CAD build for the part. Positions are in the model's coordinates, mm. A direction names the side the tool comes from. Round coordinates to 2 decimals unless told otherwise and drop trailing zeros. Loops run counter-clockwise (first coordinate to the right, second up) from the corner with the lowest first, then second, coordinate; pieces in that order, holes last.
```python
from build123d import *

# Parameters (mm, degrees)
F1_DEPTH = 17
F2_T     = 1
F3_R     = 3.5616299701
F3_R_2   = 3.3888359299
F3_R_3   = 3.7011523773
F3_R_4   = 3.561628653
F4_DEPTH = 25


with BuildPart() as f1:
    # F0 (on Top) → F1 (new body)
    with BuildSketch(Plane.XY):
        Polygon((-43.5885637999, 51.4345057309), (-45.7195602357, 49.4972355664), (-45.7195602357, -35.3551693261), (-43.7822900712, -37.6798920333), (41.6512936354, -37.6798920333), (43.5885637999, -35.5488955975), (43.5885637999, 49.303509295), (41.8450199068, 51.4345057309), align=None)
        Polygon((-9.6863470972, -24.5064590126), (-9.8800742999, -12.882841751), (7.9428050667, -12.882841751), (7.9428050667, -24.5064590126), align=None, mode=Mode.SUBTRACT)
        Polygon((-29.2527694255, 31.4806289971), (-21.6974187642, 39.2297059298), (19.7601504624, 39.4234322011), (27.315499261, 31.2869027257), (27.315499261, 10.364391841), (19.7601504624, 3.3902216237), (9.6863470972, 3.3902216237), (8.3302585408, 1.6466790112), (8.3302585408, -8.8145760819), (-9.6863470972, -8.8145760819), (-9.6863470972, 6.6835791804), (-2.3247229401, 14.4326565787), (10.4612540454, 14.4326565787), (10.4612540454, 26.2500010431), (8.5239848122, 27.9935430735), (-11.817343533, 27.9935430735), (-11.817343533, 26.4437273145), (-11.817343533, 15.0138381869), (-29.2527694255, 15.0138381869), align=None, mode=Mode.SUBTRACT)
    extrude(amount=F1_DEPTH)

    # F2
    f2_openings = [f1.faces().sort_by_distance(p)[0] for p in [
        (-0.871772, 50.172867, 17),
    ]]
    offset(amount=F2_T, openings=f2_openings, kind=Kind.INTERSECTION)

    # F3 (on Top) → F4 (cut)
    with BuildSketch(Plane.XY):
        with Locations((35.9209813178, 43.8607819378)):
            Circle(F3_R)
        with Locations((-37.6952588558, 43.4733256698)):
            Circle(F3_R_2)
        with Locations((35.9209813178, -29.5617301017)):
            Circle(F3_R_3)
        with Locations((-37.8889851272, -29.5617301017)):
            Circle(F3_R_4)
    extrude(amount=-F4_DEPTH, mode=Mode.SUBTRACT)


solid = f1.part
```
Item 1: Cut at B-B, the plane z = 4. State how many separate pieces and enclosed holes the cut face has, plus the area to 3 significant figures.
Answers follow:
separate pieces: 3
enclosed holes: 3
area: 662 mm2
Item 2: Probe line 1 (Y direction, x = 18, z = 1); line 2 (X direction, y = 0.5, z = 5.5); line 3 (Y direction, x = -29.5, z = 7.75). List the from-to ranges inside material, lowest first.
Answers follow:
line 1: y = -38.68 to -37.68, 3.39 to 4.39, 38.42 to 39.42, 51.43 to 52.43
line 2: x = -46.72 to -45.72, -9.69 to -8.69, 7.33 to 8.33, 43.59 to 44.59
line 3: y = -38.68 to -37.68, 51.43 to 52.43
Item 3: Two-plate mould, pull along X, no slides. Class faces 4 (the flat face through (14, 4.39, 8)), 5 (the flat face through (43.32, -37.33, 7.87)), 6 (the flat face through (22.89, 7.64, 7.87)), 7 (the flat face through (-12, 8, -1)): released by +X, released by -X, zero draft, split by the parting line, or undercut.
Answers follow:
face 4: undercut
face 5: released by +X
face 6: undercut
face 7: zero draft
Item 4: Cut at A-A, the plane y = 19. Give the cut face in (x, z).
Answers follow:
outline: (-46.72, -1) - (-28.25, -1) - (-28.25, 17) - (-29.25, 17) - (-29.25, 0) - (-45.72, 0) - (-45.72, 17) - (-46.72, 17) - close; (-12.82, -1) - (11.46, -1) - (11.46, 17) - (10.46, 17) - (10.46, 0) - (-11.82, 0) - (-11.82, 17) - (-12.82, 17) - close; (26.32, -1) - (44.59, -1) - (44.59, 17) - (43.59, 17) - (43.59, 0) - (27.32, 0) - (27.32, 17) - (26.32, 17) - close
Item 5: Cut at C-C, the plane y = -3. Give the cut face in (x, z), plus the area to 3 significant figures.
Answers follow:
outline: (-46.72, -1) - (-8.69, -1) - (-8.69, 17) - (-9.69, 17) - (-9.69, 0) - (-45.72, 0) - (-45.72, 17) - (-46.72, 17) - close; (7.33, -1) - (44.59, -1) - (44.59, 17) - (43.59, 17) - (43.59, 0) - (8.33, 0) - (8.33, 17) - (7.33, 17) - close
area: 143 mm2
Item 6: 3-axis set-ups, long thin cutter, end or side, ignore diameter. For faces 1 (the flat face through (0, 52.435, 8)), 2 (the flat face through (43.589, 6, 8)), 3 (the flat face through (-28.253, 23, 8)): which of +Z, -Z, +X, -X, +Y, -Y reach the whole face in a straight line?
Answers follow:
face 1: +Z, -Z, +X, -X, +Y
face 2: +Z
face 3: +Z, -Z
Item 7: Cut at D-D, the plane x = -27. Give the cut face in (y, z), plus the area to 3 significant figures.
Answers follow:
outline: (-38.68, -1) - (16.01, -1) - (16.01, 17) - (15.01, 17) - (15.01, 0) - (-37.68, 0) - (-37.68, 17) - (-38.68, 17) - close; (32.36, -1) - (52.43, -1) - (52.43, 17) - (51.43, 17) - (51.43, 0) - (33.79, 0) - (33.79, 17) - (32.36, 17) - close
area: 150 mm2
